Part model, mm, in its own coordinate system. A direction names the side the tool comes from. Round coordinates to 2 decimals unless told otherwise and drop trailing zeros. Loops run counter-clockwise (first coordinate to the right, second up) from the corner with the lowest first, then second, coordinate; pieces in that order, holes last. Notation, with made-up numbers: (-3, -23) -> (6, -23) arc R17 ccw to (6, -9) -> close; hole circle Ø2 at (58.5, 57.5). An arc over 180 degrees is marked (long way). Answer as CSV lines item,"result".
from build123d import *

# Parameters (mm, degrees)
SKETCH1_W           = 15
SKETCH1_H           = 15
BOSS_EXTRUDE1_DEPTH = 150
HOLE1_D             = 8.5
HOLE1_CBORE_D       = 14
HOLE1_CBORE_DEPTH   = 8


with BuildPart() as part:
    # Sketch1 → Boss-Extrude1 (new, symmetric)
    with BuildSketch(Plane.XY):
        Rectangle(SKETCH1_W, SKETCH1_H)
    extrude(amount=BOSS_EXTRUDE1_DEPTH, both=True)

    # Sketch3 → M8 Tapped Hole1 (revolve, cut)
    with BuildSketch(Plane(origin=(0, 0, 150), x_dir=(0, -1, 0), z_dir=(1, 0, 0))):
        Polygon((0, 0), (0, 24.292926105), (3.4, 22.25), (3.4, 0.625), (4.025, 0), align=None)
    m8_tapped_hole1 = revolve(axis=Axis((0, 0, 156.35), (0, 0, -1)), mode=Mode.SUBTRACT)

    # Mirror1: M8 Tapped Hole1 across plane
    add(m8_tapped_hole1.mirror(Plane.XY), mode=Mode.SUBTRACT)

    # Hole1 (through all)
    with Locations(Plane(origin=(0, 7.5, 0), x_dir=(1, 0, 0), z_dir=(0, 1, 0))):
        with Locations((0, 115)):
            hole1 = CounterBoreHole(HOLE1_D / 2, HOLE1_CBORE_D / 2, HOLE1_CBORE_DEPTH)

    # Mirror2: Hole1 across plane
    add(hole1.mirror(Plane.XY), mode=Mode.SUBTRACT)


solid = part.part
Q1. Two-plate mould, pull along Y, no slides. Class faces 4 (the face through (0, -7.5, 2)), 5 (the face through (0.359, 0.469, 126.062)), 6 (the face through (3.32, 0.74, -138.71)), 7 (the face through (-2.285, -4.049, -118.584)): pulls with the +Y half, pulls with the -Y half, needs draft (parallel to the pull), parting line crosses it, or undercut.
Geometry results:
face 4,"pulls with the -Y half"
face 5,"undercut"
face 6,"undercut"
face 7,"needs draft"
Q2. Saw through at A-A, the plane z = -115. Write the cut outline in (x, y), then the cut area to 3 significant figures.
Geometry results:
outline,"(-7.5, -7.5) -> (-4.25, -7.5) -> (-4.25, -0.5) -> (-7, -0.5) -> (-7, 7.5) -> (-7.5, 7.5) -> close; (4.25, -7.5) -> (7.5, -7.5) -> (7.5, 7.5) -> (7, 7.5) -> (7, -0.5) -> (4.25, -0.5) -> close"
area,"53.5 mm2"
Q3. Drill centre lines: line 1 along Z through (x, y) = (0, -5.25); line 2 along Y through (x, z) = (0, -135); line 3 along Z through (x, y) = (-1.75, 0.75). Where is each one in solid material? Low to high.
Geometry results:
line 1,"-150 to -119.25, -110.75 to 110.75, 119.25 to 150"
line 2,"-7.5 to -3.4, 3.4 to 7.5"
line 3,"-126.85 to -121.78, -108.22 to 108.22, 121.78 to 126.85"
Q4. Drop flat-ended pins along their axis: P1, Ø8, axis at x = 0, y = 0, coming from the +Z side (3 decimals); P2, Ø6, axis at x = 0, y = 0, coming from the +Z side; P3, Ø7, axis at x = 3, z = 116.5, coming from the +Y side. Give the stop position or say it passes through.
Geometry results:
P1,"z = 149.975"
P2,"z = 127.51"
P3,"y = -0.5"
Q5. Which spindle directions (+Z, -Z, +X, -X, +Y, -Y) get a long thin tool onto all of the face, cutting with end or side? Do faces 1 (the face through (6.677, 3.556, 117.103)), 2 (the face through (7.5, 0, 2)), 3 (the face through (3.32, 0.74, 138.71)). Say none if no direction does.
Geometry results:
face 1,"+Y"
face 2,"+Z, -Z, +X, +Y, -Y"
face 3,"+Z"
